Input: part model. Units: mm. Frame: model coordinates. A direction names the side the tool comes from. Give positions to 0.01 mm unless a question says otherwise; leave off trailing zeros. Loops run counter-clockwise (first coordinate to the right, second up) from the corner with the lowest first, then second, coordinate; pieces in that order, holes last. Notation, with made-up numbers: (83.5, 5) -> (91.5, 5) arc R11 cw to (91.5, 18) -> close; hole circle Ø7 at (17.5, 3). An arc over 180 degrees is marked (long way). Answer as a JSON object with one key per item and string values.
```python
from build123d import *

# Parameters (mm, degrees)
SKETCH1_W           = 42.5
SKETCH1_H           = 22.5
BOSS_EXTRUDE1_DEPTH = 13
SKETCH2_W           = 46.5
SKETCH2_H           = 26.5
BOSS_EXTRUDE2_DEPTH = 3
CUT_EXTRUDE2_REACH  = 18
SKETCH6_R           = 10.25
SKETCH7_R           = 10.25
SKETCH7_R_2         = 7.25
BOSS_EXTRUDE4_DEPTH = 3
FILLET1_R           = 2
CHAMFER1_SIZE       = 0.5


with BuildPart() as part:
    # Sketch1 → Boss-Extrude1 (new body)
    with BuildSketch(Plane.XY):
        Rectangle(SKETCH1_W, SKETCH1_H)
    extrude(amount=BOSS_EXTRUDE1_DEPTH)

    # Sketch2 → Boss-Extrude2 (add)
    with BuildSketch(Plane(origin=(0, 0, 0), x_dir=(-1, 0, 0), z_dir=(0, 0, -1))):
        Rectangle(SKETCH2_W, SKETCH2_H)
    extrude(amount=BOSS_EXTRUDE2_DEPTH)

    # Sketch6 → Cut-Extrude2 (cut, up to next)
    with BuildSketch(Plane(origin=(0, 0, -3), x_dir=(-1, 0, 0), z_dir=(0, 0, -1)), mode=Mode.PRIVATE) as cut_extrude2_sk1:
        Circle(SKETCH6_R)
    cut_extrude2_tool1 = extrude(cut_extrude2_sk1.sketch, amount=-CUT_EXTRUDE2_REACH, mode=Mode.PRIVATE) & part.part
    add(cut_extrude2_tool1.solids().sort_by_distance((0, 0, -3))[0], mode=Mode.SUBTRACT)

    # Sketch7 → Boss-Extrude4 (add)
    with BuildSketch(Plane.XY.offset(13)):
        Circle(SKETCH7_R)
        Circle(SKETCH7_R_2, mode=Mode.SUBTRACT)
    extrude(amount=-BOSS_EXTRUDE4_DEPTH)

    # Fillet1
    fillet1_edges = [part.edges().sort_by_distance(p)[0] for p in [
        (-23.25, -13.25, -1.5),
        (-23.25, 13.25, -1.5),
        (23.25, 13.25, -1.5),
        (23.25, -13.25, -1.5),
        (21.25, -11.25, 6.5),
        (-21.25, -11.25, 6.5),
        (-21.25, 11.25, 6.5),
        (21.25, 11.25, 6.5),
    ]]
    fillet(fillet1_edges, radius=FILLET1_R)

    # Chamfer1
    chamfer1_edges = [part.edges().sort_by_distance(p)[0] for p in [
        (10.25, 0, -3),
        (-7.25, 0, 13),
    ]]
    chamfer(chamfer1_edges, length=CHAMFER1_SIZE)


solid = part.part
```
Q1. Pin query (flat end, axial travel): pin 1 (2 mm diameter, centred on x = 13, z = 4, fed in from -Y); pin 2 (3 mm diameter, centred on y = -8.5, z = 11, fed in from -X); pin 3 (4 mm diameter, centred on x = -8.5, z = 2.5, fed in from +Y). Return the tip coordinate at first contact, or that it passes through.
Evaluation:
{"pin 1": "stops at y = -11.25", "pin 2": "stops at x = -21.25", "pin 3": "stops at y = 11.25"}
Q2. Ray query, line 1 along Y through (x, z) = (0, 1.5); line 2 along Y through (x, z) = (0, 11.05); line 3 along Y through (x, z) = (-15, 10.5). Return the intervals inside material, ascending.
Evaluation:
{"line 1": "y = -11.25 to -10.25, 10.25 to 11.25", "line 2": "y = -11.25 to -7.25, 7.25 to 11.25", "line 3": "y = -11.25 to 11.25"}
Q3. Section B-B, the plane z = 2.75. Return the cut outline in (x, y).
Evaluation:
{"outline": "(-21.25, -9.25) arc R2 ccw to (-19.25, -11.25) -> (19.25, -11.25) arc R2 ccw to (21.25, -9.25) -> (21.25, 9.25) arc R2 ccw to (19.25, 11.25) -> (-19.25, 11.25) arc R2 ccw to (-21.25, 9.25) -> close; hole circle Ø20.5 at (0, 0)"}
Q4. Section A-A, the plane y = 0. Return the cut outline in (x, z).
Evaluation:
{"outline": "(-23.25, -3) -> (-10.75, -3) -> (-10.25, -2.5) -> (-10.25, 10) -> (-7.25, 10) -> (-7.25, 12.5) -> (-7.75, 13) -> (-21.25, 13) -> (-21.25, 0) -> (-23.25, 0) -> close; (7.25, 10) -> (10.25, 10) -> (10.25, -2.5) -> (10.75, -3) -> (23.25, -3) -> (23.25, 0) -> (21.25, 0) -> (21.25, 13) -> (7.75, 13) -> (7.25, 12.5) -> close"}
Q5. Section D-D, the plane z = -1.5. Return the cut outline in (x, y).
Evaluation:
{"outline": "(-23.25, -11.25) arc R2 ccw to (-21.25, -13.25) -> (21.25, -13.25) arc R2 ccw to (23.25, -11.25) -> (23.25, 11.25) arc R2 ccw to (21.25, 13.25) -> (-21.25, 13.25) arc R2 ccw to (-23.25, 11.25) -> close; hole circle Ø20.5 at (0, 0)"}
Q6. Draft query along X for faces 1 (the cylindrical face through (2.222, -10.006, 3.662)), 2 (the flat face through (11, -3, -3)), 3 (the cylindrical face through (-22.68, -12.65, -1.52)), 4 (the cylindrical face through (3.35, -6.43, 11.27)). Return one class per face: +X half, -X half, draft (parallel to the pull), parting line (faces both ways), or undercut.
Evaluation:
{"face 1": "undercut", "face 2": "draft", "face 3": "-X half", "face 4": "undercut"}
Q7. Access query for faces 5 (the flat face through (-21.25, 0, 6)), 6 (the cylindrical face through (20.65, -10.68, 6.59)), 7 (the flat face through (0, 11.25, 6)), 8 (the flat face through (0, -11.25, 6)). Directions: +Z, -Z, +X, -X, +Y, -Y. A direction counts if a zero-diameter tool reaches every point of the face in a straight line with its end or side. Return the directions, or none.
Evaluation:
{"face 5": "+Z, -X, +Y, -Y", "face 6": "+Z, +X, -Y", "face 7": "+Z, +X, -X, +Y", "face 8": "+Z, +X, -X, -Y"}
Q8. Section C-C, the plane x = 0. Return the cut outline in (y, z), then the cut area to 3 significant figures.
Evaluation:
{"outline": "(-13.25, -3) -> (-10.75, -3) -> (-10.25, -2.5) -> (-10.25, 10) -> (-7.25, 10) -> (-7.25, 12.5) -> (-7.75, 13) -> (-11.25, 13) -> (-11.25, 0) -> (-13.25, 0) -> close; (7.25, 10) -> (10.25, 10) -> (10.25, -2.5) -> (10.75, -3) -> (13.25, -3) -> (13.25, 0) -> (11.25, 0) -> (11.25, 13) -> (7.75, 13) -> (7.25, 12.5) -> close", "area": "61.5 mm2"}
